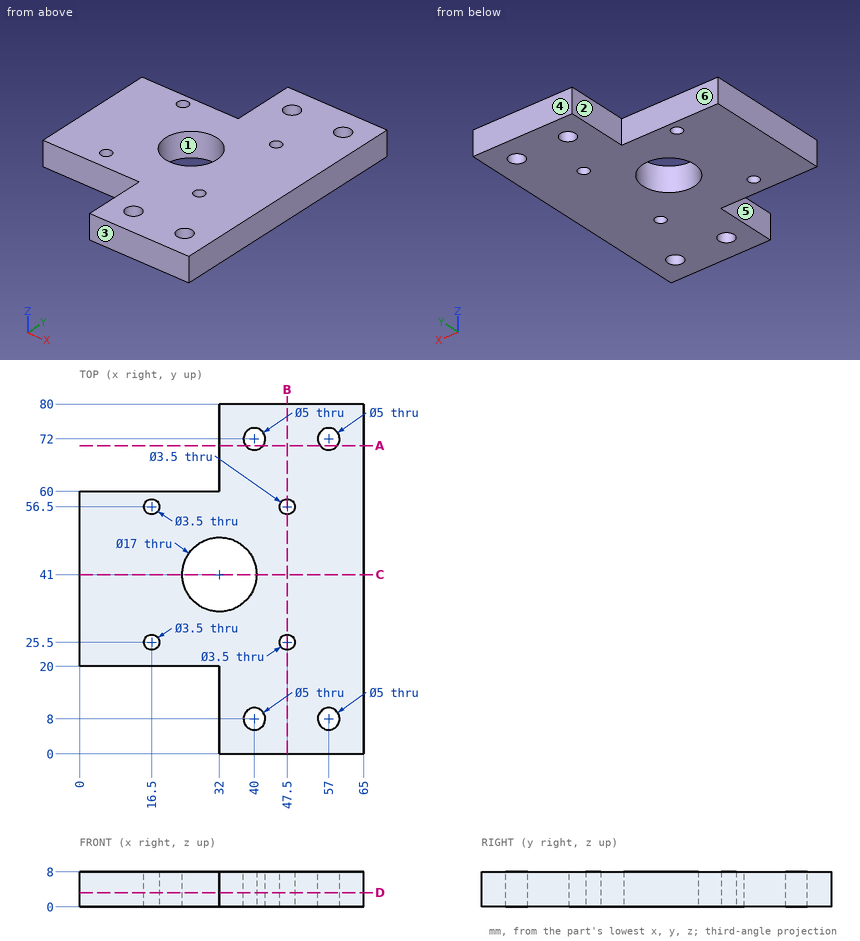
Design review of the part shown in the three views and the two pictorial views. Dimensions are in mm from the part's minimum x, y and z. A direction names the side the tool comes from. Give positions to 0.01 mm unless a question says otherwise; leave off trailing zeros. Loops run counter-clockwise (first coordinate to the right, second up) from the corner with the lowest first, then second, coordinate; pieces in that order, holes last. Notation, with made-up numbers: (66, 67.5) -> (82, 67.5) arc R13 ccw to (82, 80.5) -> close; hole circle Ø8 at (36, -1). An arc over 180 degrees is marked (long way). Put each result on its own line as item: value. Start each with the question number.
1. We need section A-A on y = 70.5. State the section outline as (x, z) points.
2. We need section D-D on z = 3.25. State how many separate pieces and enclosed holes the cut face has, then the cut area to 3 significant figures.
3. For the marked faces 4, 5 and 6, list the 3-axis set-ups (+Z, -Z, +X, -X, +Y, -Y) from which the entire face can be reached by the end or side of a thin tool; tool diameter is ignored.
4. Clearance check with flat-ended pins moving along their axes: P1, Ø4.5, axis at x = 57, y = 72, coming from the -Z side; P2, Ø4, axis at y = 73.5, z = 5.5, coming from the -X side. State where each tip first meets the part, or that it passes through.
5. We need section B-B on x = 47.5. State the section outline as (y, z) points.
6. We need section C-C on y = 41. State the section outline as (x, z) points.
7. Mouldability with a two-part tool opening along Y and no side actions: class the marked faces 1, 2 and 3 as released by +Y, released by -Y, zero draft, split by the parting line, or undercut.
8. Wall thickness on probe 1 along Y at (x, z) = (16.5, 3.75); probe 2 along X at (y, z) = (8, 5.75); probe 3 along Y at (x, z) = (47.5, 4.5): over which ranges is each line inside the solid? List them lowest first.
Determined:
1. outline: (32, 0) -> (38, 0) -> (38, 8) -> (32, 8) -> close; (42, 0) -> (55, 0) -> (55, 8) -> (42, 8) -> close; (59, 0) -> (65, 0) -> (65, 8) -> (59, 8) -> close
2. separate pieces: 1
2. enclosed holes: 9
2. area: 3,580 mm^2
3. face 4: +Z, -Z, +X, -X, +Y
3. face 5: +Z, -Z, -X, -Y
3. face 6: +Z, -Z, -X, +Y
4. P1: through
4. P2: x = 32
5. outline: (0, 0) -> (23.75, 0) -> (23.75, 8) -> (0, 8) -> close; (27.25, 0) -> (54.75, 0) -> (54.75, 8) -> (27.25, 8) -> close; (58.25, 0) -> (80, 0) -> (80, 8) -> (58.25, 8) -> close
6. outline: (0, 0) -> (23.5, 0) -> (23.5, 8) -> (0, 8) -> close; (40.5, 0) -> (65, 0) -> (65, 8) -> (40.5, 8) -> close
7. face 1: undercut
7. face 2: zero draft
7. face 3: released by -Y
8. probe 1: 20 to 23.75, 27.25 to 54.75, 58.25 to 60
8. probe 2: 32 to 37.5, 42.5 to 54.5, 59.5 to 65
8. probe 3: 0 to 23.75, 27.25 to 54.75, 58.25 to 80
